from build123d import *
from OCP.BRepFilletAPI import BRepFilletAPI_MakeChamfer

# Parameters (mm, degrees)
SKETCH3_W           = 35.4
SKETCH3_H           = 15.2
SKETCH3_R           = 2.15
SKETCH3_R_2         = 6.5
BOSS_EXTRUDE1_DEPTH = 11.55
SKETCH4_W           = 17.4
SKETCH4_H           = 15.2
SKETCH4_W_2         = 15.4
SKETCH4_H_2         = 13.2
BOSS_EXTRUDE2_DEPTH = 1
SKETCH5_W           = 9
SKETCH5_H           = 15.2
SKETCH5_R           = 2.15
BOSS_EXTRUDE3_DEPTH = 11.5
SKETCH6_R           = 4.05
CUT_EXTRUDE1_DEPTH  = 18.05
CUT_EXTRUDE4_DEPTH  = 27.033295988
CHAMFER1_SIZE       = 0.5
CHAMFER1_SIZE2      = 0.717613884
SKETCH10_W          = 5.727564928
SKETCH10_H          = 5.727564928
CUT_EXTRUDE5_DEPTH  = 0.2
CUT_EXTRUDE6_DEPTH  = 0.2


with BuildPart() as part:
    # Sketch1 → Revolve1 (revolve)
    with BuildSketch(Plane.XY, mode=Mode.PRIVATE) as revolve1_sk:
        Polygon((3.15, 0.7051349), (2.5, 0.25), (2.5, 0), (6.5, 0), (6.5, 11.55), (3.967375816, 11.55), (3.4, 9.432524629), (3.4, 7.240352815), (1.7, 6.05), (1.7, 2.55), (3.15, 2.55), align=None)
    revolve(revolve1_sk.sketch.rotate(Axis((0, 0, 0), (0, 1, 0)), 90), axis=Axis((0, 0, 0), (0, 1, 0)))

    # Sketch3 → Boss-Extrude1 (add)
    with BuildSketch(Plane.XZ):
        Rectangle(SKETCH3_W, SKETCH3_H)
        with Locations(Location((13.7, 0, 0), (0, 0, 270))):
            Circle(SKETCH3_R, mode=Mode.SUBTRACT)
        with Locations(Location((-13.7, 0, 0), (0, 0, 270))):
            Circle(SKETCH3_R, mode=Mode.SUBTRACT)
        Circle(SKETCH3_R_2, mode=Mode.SUBTRACT)
    extrude(amount=-BOSS_EXTRUDE1_DEPTH)

    # Sketch4 → Boss-Extrude2 (add)
    with BuildSketch(Plane.XZ):
        Rectangle(SKETCH4_W, SKETCH4_H)
        Rectangle(SKETCH4_W_2, SKETCH4_H_2, mode=Mode.SUBTRACT)
    extrude(amount=BOSS_EXTRUDE2_DEPTH)

    # Sketch5 → Boss-Extrude3 (add)
    with BuildSketch(Plane.XZ):
        with Locations((13.2, 0)):
            Rectangle(SKETCH5_W, SKETCH5_H)
        with Locations(Location((13.7, 0, 0), (0, 0, 270))):
            Circle(SKETCH5_R, mode=Mode.SUBTRACT)
        with Locations((-13.2, 0)):
            Rectangle(SKETCH5_W, SKETCH5_H)
        with Locations(Location((-13.7, 0, 0), (0, 0, 270))):
            Circle(SKETCH5_R, mode=Mode.SUBTRACT)
    extrude(amount=BOSS_EXTRUDE3_DEPTH)

    # Sketch6 → Cut-Extrude1 (cut)
    with BuildSketch(Plane(origin=(0, 11.55, 0), x_dir=(1, 0, 0), z_dir=(0, 1, 0))):
        with Locations((-13.7, 0)):
            Circle(SKETCH6_R)
        with Locations((13.7, 0)):
            Circle(SKETCH6_R)
    extrude(amount=-CUT_EXTRUDE1_DEPTH, mode=Mode.SUBTRACT)

    # Sketch8 → Cut-Extrude4 (cut, through all)
    with BuildSketch(Plane(origin=(0, 0, -7.6), x_dir=(-1, 0, 0), z_dir=(0, 0, -1))):
        Polygon((-17.7, -6.5), (-12.7, 11.55), (-17.7, 11.55), align=None)
        Polygon((17.7, 11.55), (17.7, -6.5), (12.7, 11.55), align=None)
    extrude(amount=-CUT_EXTRUDE4_DEPTH, mode=Mode.SUBTRACT)

    # Chamfer1: one chamfer whose edges measure the first distance from different faces: ONE call of the kernel's chamfer builder (chamfer() names one face for all edges)
    chamfer1_edges_1 = [part.edges().sort_by_distance(p)[0] for p in [
        (13.7, -11.5, 2.15),
        (17.7, -11.5, 0),
        (13.2, -11.5, -7.6),
        (8.7, -11.5, 0),
        (13.2, -11.5, 7.6),
        (-13.7, -11.5, 2.15),
        (-17.7, -11.5, 0),
        (-13.2, -11.5, 7.6),
        (-8.7, -11.5, 0),
        (-13.2, -11.5, -7.6),
        (-9.65, 11.55, 0),
        (0, 11.55, -7.6),
        (9.65, 11.55, 0),
        (0, 11.55, 7.6),
    ]]
    chamfer1_edges_2 = [part.edges().sort_by_distance(p)[0] for p in [
        (-12.7, 11.55, 5.762300945),
        (-12.7, 11.55, -5.762300945),
    ]]
    chamfer1_side_2 = [part.faces().sort_by_distance(p)[0] for p in [
        (-9.353993243, 11.55, 0),
    ]]
    chamfer1_edges_3 = [part.edges().sort_by_distance(p)[0] for p in [
        (12.7, 11.55, -5.762300945),
    ]]
    chamfer1_side_3 = [part.faces().sort_by_distance(p)[0] for p in [
        (15.4479971, 1.629730468, -5.405864047),
    ]]
    chamfer1_edges_4 = [part.edges().sort_by_distance(p)[0] for p in [
        (12.7, 11.55, 5.762300945),
    ]]
    chamfer1_side_4 = [part.faces().sort_by_distance(p)[0] for p in [
        (15.4479971, 1.629730468, 5.405864047),
    ]]
    chamfer1 = BRepFilletAPI_MakeChamfer(part.part.solid().wrapped)
    for e in chamfer1_edges_1:
        chamfer1.Add(CHAMFER1_SIZE, e.wrapped)
    for e in chamfer1_edges_2:
        chamfer1.Add(CHAMFER1_SIZE, CHAMFER1_SIZE2, e.wrapped, chamfer1_side_2[0].wrapped)  # the first distance lies on this face
    for e in chamfer1_edges_3:
        chamfer1.Add(CHAMFER1_SIZE, CHAMFER1_SIZE2, e.wrapped, chamfer1_side_3[0].wrapped)  # the first distance lies on this face
    for e in chamfer1_edges_4:
        chamfer1.Add(CHAMFER1_SIZE, CHAMFER1_SIZE2, e.wrapped, chamfer1_side_4[0].wrapped)  # the first distance lies on this face
    add(Compound.cast(chamfer1.Shape()), mode=Mode.REPLACE)

    # Sketch10 → Cut-Extrude5 (cut)
    with BuildSketch(Plane(origin=(0, -6.5, 0), x_dir=(1, 0, 0), z_dir=(0, 1, 0))):
        with Locations((-13.7, 0)):
            Rectangle(SKETCH10_W, SKETCH10_H)
        with Locations((13.7, 0)):
            Rectangle(SKETCH10_W, SKETCH10_H)
    extrude(amount=-CUT_EXTRUDE5_DEPTH, mode=Mode.SUBTRACT)

    # Sketch11 → Cut-Extrude6 (cut)
    with BuildSketch(Plane(origin=(0, -6.7, 0), x_dir=(1, 0, 0), z_dir=(0, 1, 0))):
        Polygon((-16.563782464, 0), (-13.7, -2.863782464), (-10.836217536, 0), (-13.7, 2.863782464), align=None)
        Polygon((13.7, 2.863782464), (10.836217536, 0), (13.7, -2.863782464), (16.563782464, 0), align=None)
    extrude(amount=-CUT_EXTRUDE6_DEPTH, mode=Mode.SUBTRACT)


solid = part.part
Check sheet for the modelled part. Datum: model origin and axes. Units: mm. A direction names the side the tool comes from. Round coordinates to 2 decimals unless told otherwise and drop trailing zeros. Order: outer loops, then holes, each group sorted by start corner. A loop starts at its lowest first (then second) coordinate and runs counter-clockwise, first axis right, second up. Notation, with made-up numbers: M 86,56.25 L 103,56.25 A23 cw 103,86.25 Z; hole C 29,9 d5. An arc over 180 degrees is marked long. One line per item, written item: value. Start each with the question number.
1. Section check B-B on z = 5.25. Enter the section's corners in (x, y), and give its area (3 significant figures).
2. Access from +Z, -Z, +X, -X, +Y, -Y to the whole of each face (thin tool, end or side, straight path). Record for faces 1 (the flat face through (11.4, -6.9, -0.1)), 2 (the flat face through (-11, -11.5, 2)), 3 (the flat face through (-0.1, -0.5, 6.6)).
3. Scan lines: line 1 along X through (y, z) = (-9.5, 0); line 2 along X through (y, z) = (-9, -1.25); line 3 along Z through (x, y) = (13.7, -2). Record each from-to range of solid material in increasing order.
4. Release check for a two-part mould opening along Z. For faces 4 (the cylindrical face through (-11.57, -8.82, 0.28)), 5 (the flat face through (11, -11.5, 2)), 6 (the flat face through (-16, -6.9, 0)) record: released by +Z, released by -Z, zero draft, split by the parting line, or undercut.
5. Section check A-A on y = -8.25. Enter the section's corners in (x, z).
6. Gauge pin test, flat ends, axial feed: P1, Ø0.7, axis at x = 13.5, z = -2, coming from the +Y side; P2, Ø1.2, axis at x = 17, z = 0.5, coming from the +Y side; P3, Ø4, axis at y = 2, z = 4, coming from the +X side. Record the tip position at first contact, or that the pin passes through.
Results found:
1. outline: M -17.7,-11 L -17.2,-11.5 L -9.2,-11.5 L -8.7,-11 L -8.7,-1 L -7.7,-1 L -7.7,0 L 7.7,0 L 7.7,-1 L 8.7,-1 L 8.7,-11 L 9.2,-11.5 L 17.2,-11.5 L 17.7,-11 L 17.7,-6.5 L 12.83,11.07 L 11.98,11.55 L -12.2,11.55 L -12.89,10.86 L -17.7,-6.5 Z
1. area: 527 mm^2
2. face 1: +Y
2. face 2: +Z, -Z, +X, -X, -Y
2. face 3: -Y
3. line 1: -17.7 to -15.85, -11.55 to -8.7, 8.7 to 11.55, 15.85 to 17.7
3. line 2: -17.7 to -15.45, -11.95 to -8.7, 8.7 to 11.95, 15.45 to 17.7
3. line 3: -7.6 to -4.05, 4.05 to 7.6
4. face 4: undercut
4. face 5: zero draft
4. face 6: undercut
5. outline: M -17.7,-7.6 L -8.7,-7.6 L -8.7,7.6 L -17.7,7.6 Z; M 8.7,-7.6 L 17.7,-7.6 L 17.7,7.6 L 8.7,7.6 Z; hole C -13.7,0 d4.3; hole C 13.7,0 d4.3
6. P1: y = -6.9
6. P2: y = -6.5
6. P3: x = 15.9
